Input: dimensioned drawing with shaded views. Units: mm. Origin: part minimum x, y, z. Round coordinates to 2 decimals unless told otherwise and drop trailing zeros. Loops run counter-clockwise (first coordinate to the right, second up) from the corner with the lowest first, then second, coordinate; pieces in that order, holes last. Notation, with made-up numbers: (-10, 51) - (0, 51) arc R31 cw to (0, 86) - close; hole circle Ø3 at (82.25, -23). An arc over 180 degrees is marked (long way). One line per question, with ' | ' between items. Start each with the question number.
1. Cut plane A-A (x = 50.8). Return loops of the section in (y, z) (1 decimal), then the cut area to 3 significant figures.
2. Cut plane B-B (y = 88). Return loops of the section in (x, z).
3. Ray query, line 1 (Y direction, x = 50.8, z = 5.75) (1 decimal); line 2 (X direction, y = 3, z = 6); line 3 (X direction, y = 10, z = 7.75) (1 decimal). Return the intervals inside material, ascending.
4. Mould query, pull axis X, two halves, no side actions, for the marked faces 1 and 2. Classes: pulls with the +X half, pulls with the -X half, needs draft (parallel to the pull), parting line crosses it, or undercut.
5. Cut plane C-C (z = 5.75). State how many separate pieces and enclosed holes the cut face has, then the cut area to 3 significant figures.
6. Pin query (flat end, axial travel): pin 1 (1.4 mm diameter, centred on x = 18, z = 5.5, fed in from -Y). Return the tip coordinate at first contact, or that it passes through.
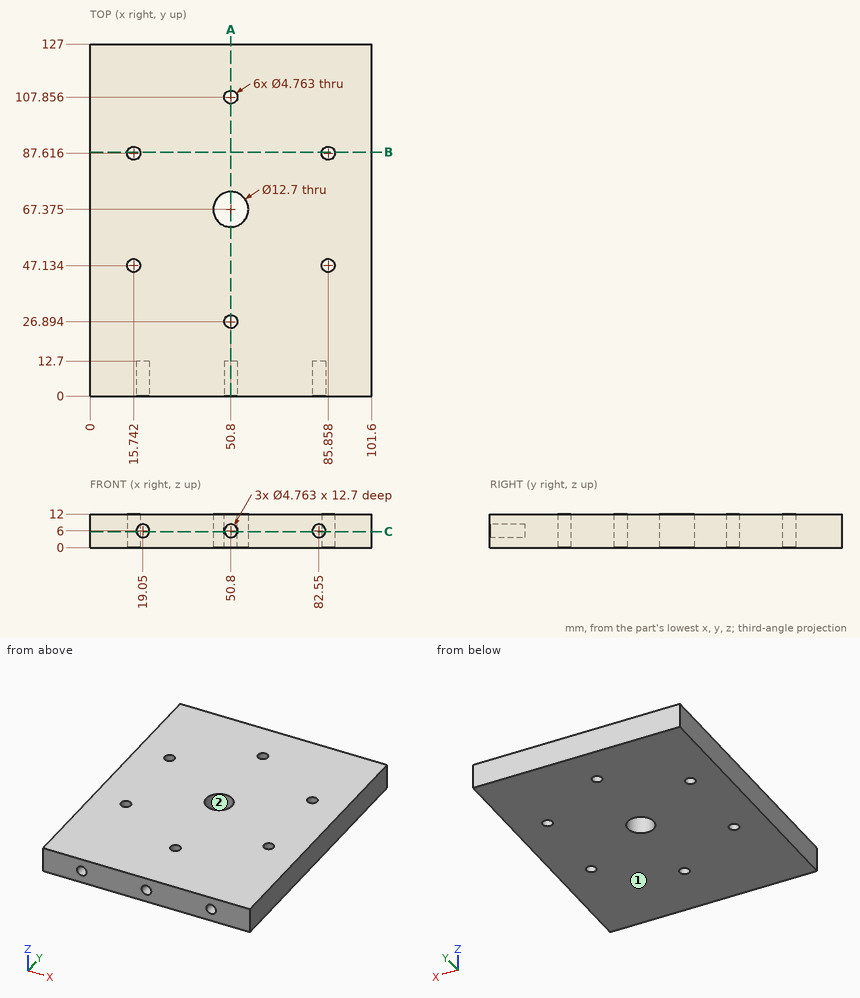
Answers follow:
1) outline: (0, 0) - (24.5, 0) - (24.5, 12) - (0, 12) - (0, 8.4) - (12.7, 8.4) - (12.7, 3.6) - (0, 3.6) - close; (29.3, 0) - (61, 0) - (61, 12) - (29.3, 12) - close; (73.7, 0) - (105.5, 0) - (105.5, 12) - (73.7, 12) - close; (110.2, 0) - (127, 0) - (127, 12) - (110.2, 12) - close | area: 1,200 mm2
2) outline: (0, 0) - (13.39, 0) - (13.39, 12) - (0, 12) - close; (18.09, 0) - (83.51, 0) - (83.51, 12) - (18.09, 12) - close; (88.21, 0) - (101.6, 0) - (101.6, 12) - (88.21, 12) - close
3) line 1: y = 12.7 to 24.5, 29.3 to 61, 73.7 to 105.5, 110.2 to 127 | line 2: x = 0 to 16.67, 21.43 to 48.42, 53.18 to 80.17, 84.93 to 101.6 | line 3: x = 0 to 17.4, 20.7 to 49.2, 52.4 to 80.9, 84.2 to 101.6
4) face 1: needs draft | face 2: undercut
5) separate pieces: 1 | enclosed holes: 7 | area: 12,500 mm2
6) pin 1: stops at y = 12.7
